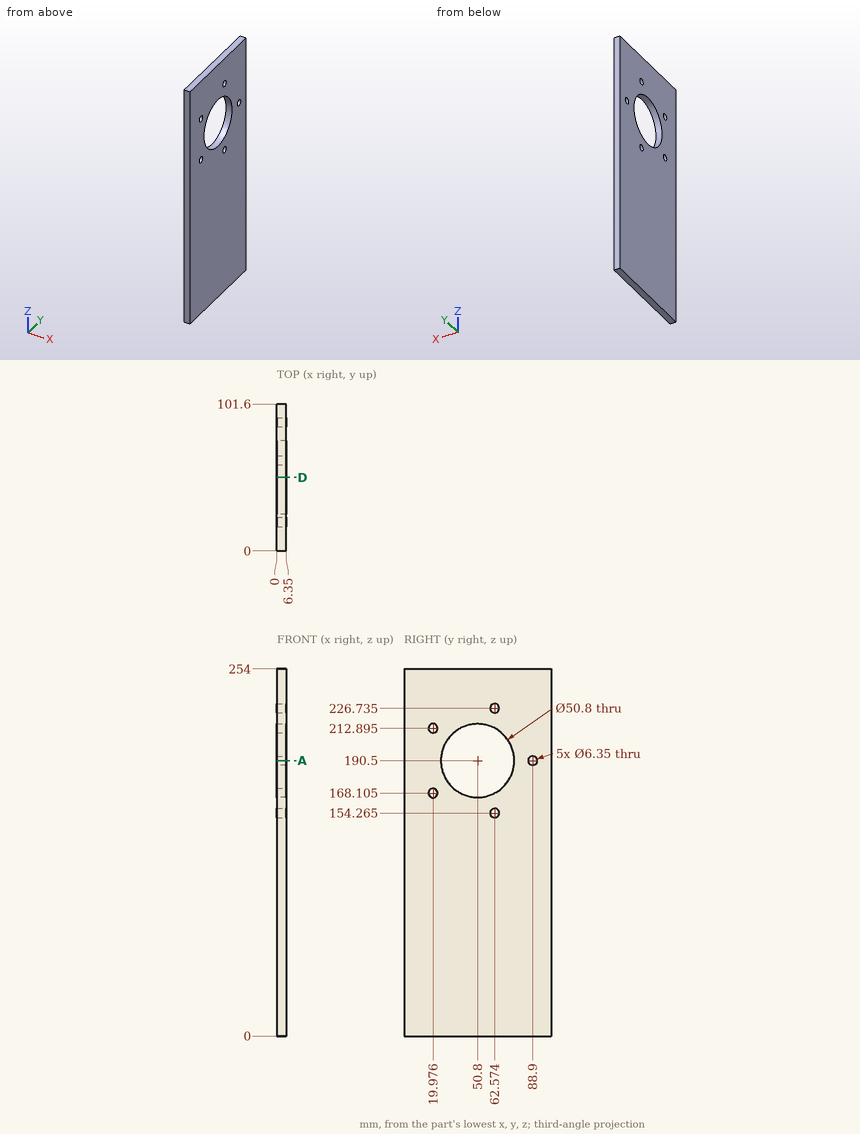
Here's the drawing with two shaded views (mm, measured from the low corner). I have some questions. Round coordinates to 2 decimals unless told otherwise and drop trailing zeros. Order: outer loops, then holes, each group sorted by start corner. A loop starts at its lowest first (then second) coordinate and runs counter-clockwise, first axis right, second up. Notation, with made-up numbers: (62, 86) -> (79, 86) arc R24 cw to (79, 122) -> close; hole circle Ø9 at (81, 53.5). An arc over 180 degrees is marked (long way). Write each question's results on one line, items separated by ' | '. Start each with the question number.
Item 1: Will this pin go through, and if not, where does the flat tip stop? pin 1 (5 mm diameter, centred on y = 19.98, z = 168.11, fed in from +X).
Item 2: Please list where these lines run through material, in increasing order: L1, parallel to Z at x = 2, y = 20.5 (1 decimal); L2, parallel to Y at x = 4, z = 190.5 (1 decimal); L3, parallel to Z at x = 3.25, y = 65 (1 decimal).
Item 3: If we section it at A-A, the plane z = 190.5: State how many separate pieces and enclosed holes the cut face has, then the cut area to 3 significant figures.
Item 4: If we section it at D-D, the plane y = 50.8: Write out the boundary of the cut face in (x, z), then the cut area to 3 significant figures.
Results:
1) pin 1: passes through
2) L1: z = 0 to 165, 171.2 to 209.8, 216 to 254 | L2: y = 0 to 25.4, 76.2 to 85.7, 92.1 to 101.6 | L3: z = 0 to 152.2, 156.3 to 169.4, 211.6 to 224.7, 228.8 to 254
3) separate pieces: 3 | enclosed holes: 0 | area: 282 mm2
4) outline: (0, 0) -> (6.35, 0) -> (6.35, 165.1) -> (0, 165.1) -> close; (0, 215.9) -> (6.35, 215.9) -> (6.35, 254) -> (0, 254) -> close | area: 1,290 mm2
